```python
from build123d import *

# Parameters (mm, degrees)
SKETCH1_W                                            = 120
SKETCH1_H                                            = 50
MAIN_DEPTH                                           = 10
SKETCH2_R                                            = 1.5
LINEAR_BEARING_MOUNT_DEPTH                           = 11
SKETCH5_R                                            = 3.5
LINEAR_BEARING_COUNTERSINK_DEPTH                     = 4
SKETCH6_R                                            = 2.5
CUT_EXTRUDE1_DEPTH                                   = 11
CSK_FOR_M5_SOCKET_COUNTERSUNK_HEAD_SCREW_D           = 5.5
CSK_FOR_M5_SOCKET_COUNTERSUNK_HEAD_SCREW_DEPTH       = 10
CSK_FOR_M5_SOCKET_COUNTERSUNK_HEAD_SCREW_CSINK_D     = 11.47
CSK_FOR_M5_SOCKET_COUNTERSUNK_HEAD_SCREW_CSINK_ANGLE = 90
CSK_FOR_M5_SOCKET_COUNTERSUNK_HEAD_SCREW_TIP         = 1.652366702


with BuildPart() as part:
    # Sketch1 → main (new body)
    with BuildSketch(Plane(origin=(0, 0, 0), x_dir=(1, 0, 0), z_dir=(0, 1, 0))):
        Rectangle(SKETCH1_W, SKETCH1_H)
    extrude(amount=MAIN_DEPTH)

    # Sketch2 → linear_bearing_mount (cut, through all)
    with BuildSketch(Plane(origin=(0, 10, 0), x_dir=(1, 0, 0), z_dir=(0, 1, 0))):
        with Locations((-28, -12)):
            Circle(SKETCH2_R)
        with Locations((-46, -12)):
            Circle(SKETCH2_R)
        with Locations((28, -12)):
            Circle(SKETCH2_R)
        with Locations((46, -12)):
            Circle(SKETCH2_R)
        with Locations((46, 12)):
            Circle(SKETCH2_R)
        with Locations((28, 12)):
            Circle(SKETCH2_R)
        with Locations((-46, 12)):
            Circle(SKETCH2_R)
        with Locations((-28, 12)):
            Circle(SKETCH2_R)
    extrude(amount=-LINEAR_BEARING_MOUNT_DEPTH, mode=Mode.SUBTRACT)

    # Sketch5 → linear_bearing_countersink (cut)
    with BuildSketch(Plane(origin=(0, 10, 0), x_dir=(1, 0, 0), z_dir=(0, 1, 0))):
        with Locations((-46, 12)):
            Circle(SKETCH5_R)
        with Locations((-28, 12)):
            Circle(SKETCH5_R)
        with Locations((-28, -12)):
            Circle(SKETCH5_R)
        with Locations((-46, -12)):
            Circle(SKETCH5_R)
        with Locations((46, -12)):
            Circle(SKETCH5_R)
        with Locations((28, -12)):
            Circle(SKETCH5_R)
        with Locations((28, 12)):
            Circle(SKETCH5_R)
        with Locations((46, 12)):
            Circle(SKETCH5_R)
    extrude(amount=-LINEAR_BEARING_COUNTERSINK_DEPTH, mode=Mode.SUBTRACT)

    # Sketch6 → Cut-Extrude1 (cut, through all)
    with BuildSketch(Plane.XZ):
        with Locations((-50, 0)):
            Circle(SKETCH6_R)
        with Locations((-30, 0)):
            Circle(SKETCH6_R)
        with Locations((-10, 0)):
            Circle(SKETCH6_R)
        with Locations((10, 0)):
            Circle(SKETCH6_R)
        with Locations((30, 0)):
            Circle(SKETCH6_R)
        with Locations((50, 0)):
            Circle(SKETCH6_R)
    extrude(amount=-CUT_EXTRUDE1_DEPTH, mode=Mode.SUBTRACT)

    # CSK for M5 socket countersunk head screw1
    with Locations(Plane(origin=(0, 0, 0), x_dir=(-1, 0, 0), z_dir=(0, -1, 0))):
        with Locations((-50, 0), (-30, 0), (-10, 0), (10, 0), (30, 0), (50, 0)):
            CounterSinkHole(CSK_FOR_M5_SOCKET_COUNTERSUNK_HEAD_SCREW_D / 2, CSK_FOR_M5_SOCKET_COUNTERSUNK_HEAD_SCREW_CSINK_D / 2, depth=CSK_FOR_M5_SOCKET_COUNTERSUNK_HEAD_SCREW_DEPTH, counter_sink_angle=CSK_FOR_M5_SOCKET_COUNTERSUNK_HEAD_SCREW_CSINK_ANGLE)
            with Locations((0, 0, -(CSK_FOR_M5_SOCKET_COUNTERSUNK_HEAD_SCREW_DEPTH + CSK_FOR_M5_SOCKET_COUNTERSUNK_HEAD_SCREW_TIP / 2))):  # 118° drill point
                Cone(0, CSK_FOR_M5_SOCKET_COUNTERSUNK_HEAD_SCREW_D / 2, CSK_FOR_M5_SOCKET_COUNTERSUNK_HEAD_SCREW_TIP, mode=Mode.SUBTRACT)


solid = part.part
```
CAD build for the part. Positions are in the model's coordinates, mm. A direction names the side the tool comes from. Round coordinates to 2 decimals unless told otherwise and drop trailing zeros. One line per question, with ' | ' between items.
1. Mould opens along Z. For faces 1 (the flat face through (-1, 5, 25)), 2 (the cylindrical face through (-7.46, 6.54, 1.05)), 3 (the flat face through (-1, 0, 0)) say: pulls with the +Z half, pulls with the -Z half, needs draft (parallel to the pull), parting line crosses it, or undercut.
Working result:
face 1: pulls with the +Z half | face 2: undercut | face 3: needs draft
2. Which spindle directions (+Z, -Z, +X, -X, +Y, -Y) get a long thin tool onto all of the face, cutting with end or side? Do faces 4 (the cylindrical face through (29.615, 8.028, -8.895)), 5 (the cylindrical face through (-47.5, 3.04, -12.07)). Say none if no direction does.
Working result:
face 4: +Y | face 5: +Y, -Y
3. Probe L1, parallel to X at y = 7.8, z = 12; L2, parallel to Z at x = 46, y = 9; L3, parallel to X at y = 1.9, z = -12. List the from-to ranges inside material, lowest first. Write a range as from..to.
Working result:
L1: -60..-49.5, -42.5..-31.5, -24.5..24.5, 31.5..42.5, 49.5..60 | L2: -25..-15.5, -8.5..8.5, 15.5..25 | L3: -60..-47.5, -44.5..-29.5, -26.5..26.5, 29.5..44.5, 47.5..60
4. Cut at A-A on y = 7.5. Count the separate pieces of the cut face and the enclosed holes in it, and give its area (3 significant figures).
Working result:
separate pieces: 1 | enclosed holes: 14 | area: 5,550 mm2
5. Pin check, flat tips, straight feed: pin 1 Ø6.5 at (x, z) = (10, 0) entering from -Y (3 decimals); pin 2 Ø5 at (x, z) = (-46, 12) entering from +Y; pin 3 Ø1.8 at (x, z) = (28, -12) entering from -Y. Stop position of each tip, or through.
Working result:
pin 1: y = 2.485 | pin 2: y = 6 | pin 3: through
